Geometry: final body of the model. Coordinates: model frame, mm. Face numbers are marked on the shaded views. Round coordinates to 2 decimals unless told otherwise and drop trailing zeros. Loops run counter-clockwise (first coordinate to the right, second up) from the corner with the lowest first, then second, coordinate; pieces in that order, holes last. Notation, with made-up numbers: (-3, -23) - (16, -23) arc R32 ccw to (16, 11) - close; hole circle Ø6 at (62.25, 66). An arc over 180 degrees is marked (long way). Return JSON: item names as keys, results as strings. Group by question number.
1. First-contact query: pin 1 Ø1.5 at (x, y) = (7.5, -8) entering from -Z; pin 2 Ø3 at (x, z) = (3.5, 4.5) entering from -Y. Flat tips, straight axial feed; report the tip coordinate or a pass-through.
2. Section B-B on z = 0. Return loops of the section in (x, y).
3. Section D-D on y = 0. Return loops of the section in (x, z), and give its area (3 significant figures).
4. Section A-A on x = 0. Return loops of the section in (y, z).
5. Draft query along Y for the marked faces 1, 2 and 3. Return one class per face: +Y half, -Y half, draft (parallel to the pull), parting line (faces both ways), or undercut.
6. Section C-C on y = 5.25. Return loops of the section in (x, z), and give its area (3 significant figures).
7. Material intervals for probe 1 along X at (y, z) = (-7, -0.25); probe 2 along Y at (x, z) = (0, 8.35), sorted ascending.
from build123d import *

# Parameters (mm, degrees)
F0_W           = 25.4
F0_H           = 25.4
F0_R           = 6.793342
F1_DEPTH       = 12.7
F2_R           = 6.35
F4_D           = 3.175
F4_DEPTH       = 12.7
F4_CSINK_D     = 7.62
F4_CSINK_ANGLE = 90


with BuildPart() as f1:
    # F0 (on Front) → F1 (new body, symmetric)
    with BuildSketch(Plane.XZ):
        Rectangle(F0_W, F0_H)
        Circle(F0_R, mode=Mode.SUBTRACT)
    extrude(amount=F1_DEPTH, both=True)

    # F2
    f2_edges = [f1.edges().sort_by_distance(p)[0] for p in [
        (12.7, 0, 12.7),
        (-12.7, 0, 12.7),
        (-12.7, 0, -12.7),
        (12.7, 0, -12.7),
    ]]
    fillet(f2_edges, radius=F2_R)

    # F4
    with Locations(Plane.XY.offset(12.7)):
        with Locations((0, 0)):
            CounterSinkHole(F4_D / 2, F4_CSINK_D / 2, depth=F4_DEPTH, counter_sink_angle=F4_CSINK_ANGLE)


solid = f1.part
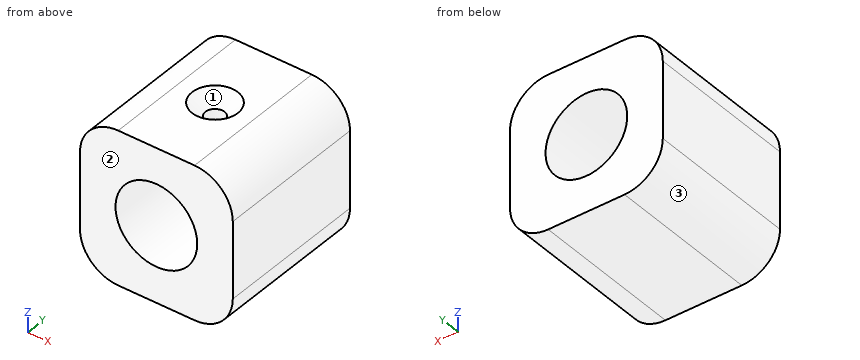
Taken from the geometry:
{
 "1": {"pin 1": "z = -12.69", "pin 2": "y = -12.7"},
 "2": {"outline": "(-12.7, -12.7) - (-6.79, -12.7) - (-6.79, 12.7) - (-12.7, 12.7) - close; (6.79, -12.7) - (12.7, -12.7) - (12.7, 12.7) - (6.79, 12.7) - close"},
 "3": {"outline": "(-12.7, -6.35) arc R6.35 ccw to (-6.35, -12.7) - (6.35, -12.7) arc R6.35 ccw to (12.7, -6.35) - (12.7, 6.35) arc R6.35 ccw to (6.35, 12.7) - (3.81, 12.7) - (1.59, 10.48) - (1.59, 6.61) arc R6.79 cw (long way) to (-1.59, 6.61) - (-1.59, 10.48) - (-3.81, 12.7) - (-6.35, 12.7) arc R6.35 ccw to (-12.7, 6.35) - close", "area": "442 mm2"},
 "4": {"outline": "(-12.7, -12.7) - (12.7, -12.7) - (12.7, -6.79) - (-12.7, -6.79) - close; (-12.7, 6.79) - (-1.59, 6.79) - (-1.59, 10.48) - (-3.81, 12.7) - (-12.7, 12.7) - close; (1.59, 6.79) - (12.7, 6.79) - (12.7, 12.7) - (3.81, 12.7) - (1.59, 10.48) - close"},
 "5": {"face 1": "undercut", "face 2": "-Y half", "face 3": "draft"},
 "6": {"outline": "(-12.7, -6.35) arc R6.35 ccw to (-6.35, -12.7) - (6.35, -12.7) arc R6.35 ccw to (12.7, -6.35) - (12.7, 6.35) arc R6.35 ccw to (6.35, 12.7) - (-6.35, 12.7) arc R6.35 ccw to (-12.7, 6.35) - close; hole circle Ø13.59 at (0, 0)", "area": "466 mm2"},
 "7": {"probe 1": "-12.7 to -6.79, 6.79 to 12.7", "probe 2": "-12.7 to -1.59, 1.59 to 12.7"}
}
